Model file for the job. Use its own axes, mm. Face numbers are marked on the shaded views. A direction names the side the tool comes from. Coordinates: 2 decimals unless noted, no trailing zeros. Write each loop counter-clockwise with the first axis right and the second up, starting at its lowest first coordinate (ties: lowest second). Pieces come first, ordered by that corner, then holes. Notation, with made-up numbers: (50, -39) - (85, -39) arc R16 cw to (85, -26) - close; hole circle Ø3 at (54.25, 60). An arc over 180 degrees is marked (long way). Put each result on its own line as item: value. Start each with the question number.
1. Drill centre lines: L1, parallel to Y at x = 0, z = 1.7; L2, parallel to Z at x = 7, y = -6.25; L3, parallel to Z at x = 6.75, y = -4.5. Where is each one in solid material? Low to high. Write a range as from..to.
2. Pull direction Z, two halves, no side cores. Call the marked faces 3, 4, 5 and 6: released by +Z, released by -Z, zero draft, split by the parting line, or undercut.
3. Which spindle directions (+Z, -Z, +X, -X, +Y, -Y) get a long thin tool onto all of the face, cutting with end or side? Do the marked faces 1 and 2. Say none if no direction does.
4. Saw through at C-C, the plane z = 0.5. Write the cut outline in (x, y).
5. Saw through at A-A, the plane x = 0. Write the cut outline in (y, z), plus the area to 3 significant figures.
6. Drop flat-ended pins along their axis: P1, Ø6, axis at y = 0.5, z = -4, coming from the -X side; P2, Ø8, axis at x = -6.5, y = 5.5, coming from the +Z side; P3, Ø4, axis at x = -2.5, y = -0.5, coming from the -Z side. Give the stop position or say it passes through.
7. Saw through at D-D, the plane y = 5.75. Write the cut outline in (x, z), plus the area to 3 significant figures.
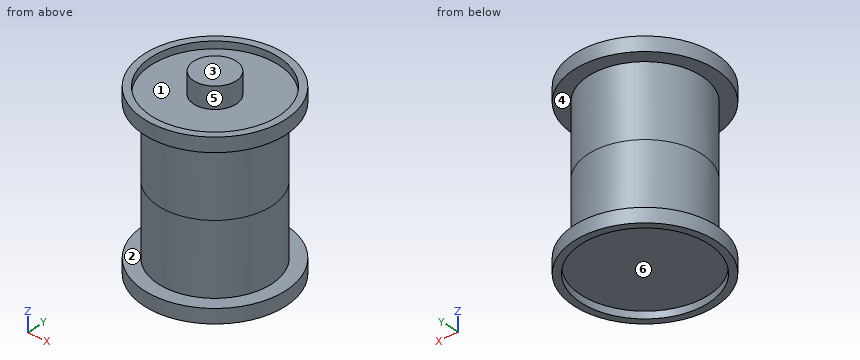
```python
from build123d import *

# Parameters (mm, degrees)
CROQUIS1_R     = 10
EXTRUIR1_DEPTH = 2
VACIADO1_T     = -1
CROQUIS2_R     = 8
EXTRUIR2_DEPTH = 10
CROQUIS4_R     = 3
EXTRUIR4_DEPTH = 3


with BuildPart() as part:
    # Croquis1 → Extruir1 (new body)
    with BuildSketch(Plane.XY):
        Circle(CROQUIS1_R)
    extrude(amount=EXTRUIR1_DEPTH)

    # Vaciado1
    vaciado1_openings = [part.faces().sort_by_distance(p)[0] for p in [
        (0, 0, 2),
    ]]
    offset(amount=VACIADO1_T, openings=vaciado1_openings, kind=Kind.INTERSECTION)

    # Croquis2 → Extruir2 (add)
    with BuildSketch(Plane(origin=(0, 0, 0), x_dir=(-1, 0, 0), z_dir=(0, 0, -1))):
        with Locations(Location((0, 0, 0), (0, 0, 180))):  # turned: the seam where the file's is
            Circle(CROQUIS2_R)
    extrude(amount=EXTRUIR2_DEPTH)

    # Simetría3: part across plane


with BuildPart() as part_1:
    add(part.part)
    add(part.part.mirror(Plane(origin=(0, 0, -10), x_dir=(1, 0, 0), z_dir=(0, 0, -1))))

    # Croquis4 → Extruir4 (add)
    with BuildSketch(Plane.XY.offset(1)):
        Circle(CROQUIS4_R)
    extrude(amount=EXTRUIR4_DEPTH)


solid = part_1.part
```
Final values:
1. L1: y = -10..-9, -3..3, 9..10
1. L2: z = -22..-20, 0..2
1. L3: z = -21..-20, 0..1
2. face 3: released by +Z
2. face 4: undercut
2. face 5: zero draft
2. face 6: released by -Z
3. face 1: +Z
3. face 2: none
4. outline: circle Ø20 at (0, 0)
5. outline: (-10, -22) - (-9, -22) - (-9, -21) - (9, -21) - (9, -22) - (10, -22) - (10, -20) - (8, -20) - (8, 0) - (10, 0) - (10, 2) - (9, 2) - (9, 1) - (3, 1) - (3, 4) - (-3, 4) - (-3, 1) - (-9, 1) - (-9, 2) - (-10, 2) - (-10, 0) - (-8, 0) - (-8, -20) - (-10, -20) - close
5. area: 382 mm²
6. P1: stops at x = -8
6. P2: stops at z = 2
6. P3: stops at z = -21
7. outline: (-8.18, -22) - (-6.92, -22) - (-6.92, -21) - (6.92, -21) - (6.92, -22) - (8.18, -22) - (8.18, -20) - (5.56, -20) - (5.56, 0) - (8.18, 0) - (8.18, 2) - (6.92, 2) - (6.92, 1) - (-6.92, 1) - (-6.92, 2) - (-8.18, 2) - (-8.18, 0) - (-5.56, 0) - (-5.56, -20) - (-8.18, -20) - close
7. area: 260 mm²
